from build123d import *

# Parameters (mm, degrees)
SKETCH_W     = 26
SKETCH_H     = 8
SKETCH_R     = 1.7
PAD_DEPTH    = 5
SKETCH002_R  = 4
POCKET_DEPTH = 8.001
SKETCH003_W  = 6.25
SKETCH003_H  = 8
SKETCH003_R  = 1.7
PAD001_DEPTH = 6


with BuildPart() as part:
    # Sketch → Pad (new body)
    with BuildSketch(Plane.XY):
        with Locations((10, 0)):
            Rectangle(SKETCH_W, SKETCH_H)
        Circle(SKETCH_R, mode=Mode.SUBTRACT)
        with Locations((20, 0)):
            Circle(SKETCH_R, mode=Mode.SUBTRACT)
    extrude(amount=PAD_DEPTH)

    # Sketch002 → Pocket (cut, through all)
    with BuildSketch(Plane.XZ.offset(4)):
        with Locations((10, -1)):
            Circle(SKETCH002_R)
    extrude(amount=-POCKET_DEPTH, mode=Mode.SUBTRACT)

    # Sketch003 → Pad001 (new body)
    with BuildSketch(Plane.XY.offset(5)):
        with Locations((0.125, 0)):
            Rectangle(SKETCH003_W, SKETCH003_H)
        Circle(SKETCH003_R, mode=Mode.SUBTRACT)
        with Locations((19.875, 0)):
            Rectangle(SKETCH003_W, SKETCH003_H)
        with Locations((20, 0)):
            Circle(SKETCH003_R, mode=Mode.SUBTRACT)
    extrude(amount=PAD001_DEPTH)


solid = part.part
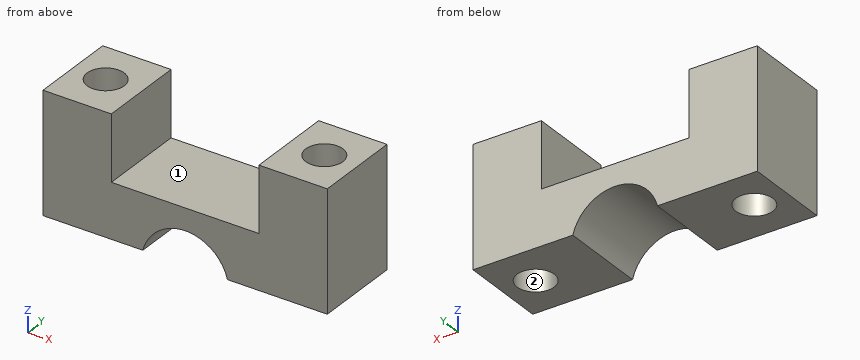
The listing builds one solid part. Answer for the finished solid, in the listing's coordinates (mm). Face numbers are marked on the shaded views. A direction names the side the tool comes from. Coordinates: 2 decimals unless noted, no trailing zeros. Loops run counter-clockwise (first coordinate to the right, second up) from the corner with the lowest first, then second, coordinate; pieces in that order, holes last. Notation, with made-up numbers: (89.25, -12) -> (96.25, -12) arc R24 cw to (96.25, 11) -> close; hole circle Ø1 at (-12.75, 15.25). An arc over 180 degrees is marked (long way). Answer in a Markdown table with one row per item. Add a question column.
1. The part is cut by section D-D, the plane y = 3.5. Write down the section's boundary in (x, z).
2. The part is cut by section B-B, the plane y = 0. Write down the section's boundary in (x, z).
3. The part is cut by section A-A, the plane z = 7.5. Write down the section's boundary in (x, y).
4. Consider line 1 (Y direction, x = 0, z = 3); line 2 (X direction, y = -2.5, z = 6.25); line 3 (X direction, y = 0.25, z = 6). Determine where each line is inside the solid, lowest interval first. Write a range as [from, to].
5. For the marked faces 1 and 2, determine the directions among +Z, -Z, +X, -X, +Y, -Y from which every point of the face is accessible in a straight line to the end or side of a thin tool.
6. A flat-ended cylindrical pin translates along its axis: P1, Ø2, axis at x = 9, y = -3, coming from the -Z side. Find the tip coordinate at first contact, or state that the pin passes through.
7. The part is cut by section C-C, the plane x = 20. Write down the section's boundary in (y, z), then the cut area to 3 significant figures.
Answer below:
| question | item | result |
|---|---|---|
| 1 | outline | (-3, 0) -> (6.13, 0) arc R4 cw to (13.87, 0) -> (23, 0) -> (23, 11) -> (16.75, 11) -> (16.75, 5) -> (3.25, 5) -> (3.25, 11) -> (-3, 11) -> close |
| 2 | outline | (-3, 0) -> (-1.7, 0) -> (-1.7, 11) -> (-3, 11) -> close; (1.7, 0) -> (6.13, 0) arc R4 cw to (13.87, 0) -> (18.3, 0) -> (18.3, 11) -> (16.75, 11) -> (16.75, 5) -> (3.25, 5) -> (3.25, 11) -> (1.7, 11) -> close; (21.7, 0) -> (23, 0) -> (23, 11) -> (21.7, 11) -> close |
| 3 | outline | (-3, -4) -> (3.25, -4) -> (3.25, 4) -> (-3, 4) -> close; (16.75, -4) -> (23, -4) -> (23, 4) -> (16.75, 4) -> close; hole circle Ø3.4 at (0, 0); hole circle Ø3.4 at (20, 0) |
| 4 | line 1 | [-4, -1.7], [1.7, 4] |
| 4 | line 2 | [-3, 3.25], [16.75, 23] |
| 4 | line 3 | [-3, -1.68], [1.68, 3.25], [16.75, 18.32], [21.68, 23] |
| 5 | face 1 | +Z, +Y, -Y |
| 5 | face 2 | +Z, -Z |
| 6 | P1 | z = 2.46 |
| 7 | outline | (-4, 0) -> (-1.7, 0) -> (-1.7, 11) -> (-4, 11) -> close; (1.7, 0) -> (4, 0) -> (4, 11) -> (1.7, 11) -> close |
| 7 | area | 50.6 mm2 |
